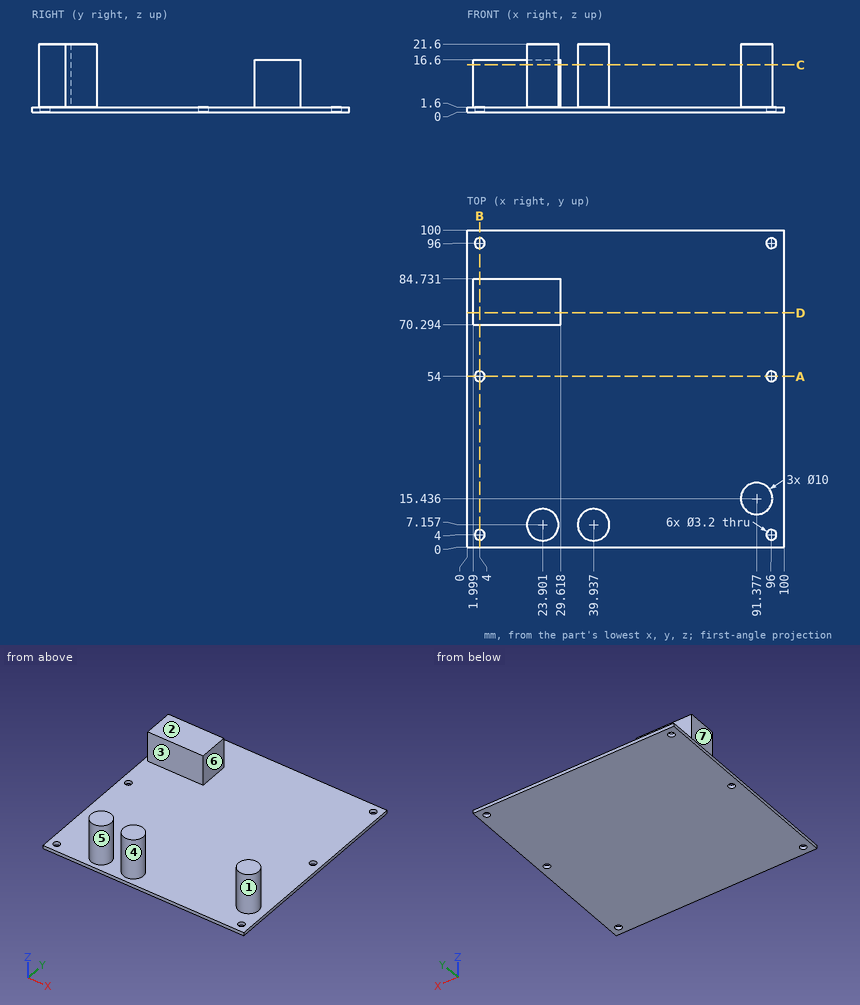
Study the drawing (mm; zero at the part's minimum x, y, z) and answer. A direction names the side the tool comes from. Round coordinates to 2 decimals unless told otherwise and drop trailing zeros. Write each loop counter-clockwise with the first axis right and the second up, starting at its lowest first coordinate (ties: lowest second). Pieces come first, ordered by that corner, then holes. Notation, with made-up numbers: (85, 68.25) - (131, 68.25) arc R3 ccw to (131, 73.25) - close; hole circle Ø8 at (-23, 49.5). An arc over 180 degrees is marked (long way). Return JSON: item names as keys, results as strings. Group by question number.
Q1. Find the intervals of material crossed by L1, parallel to Y at x = 96, z = 0.7; L2, parallel to Z at x = 7.5, y = 47; L3, parallel to Z at x = 21, y = 77, in increasing order.
Q2. Each of these flat-tipped pins is pushed along its axis until it touches: pin 1 Ø4 at (y, z) = (79.5, 5.5) entering from -X; pin 2 Ø12 at (x, z) = (31.5, 18.5) entering from -Y; pin 3 Ø4.5 at (x, z) = (12.5, 6) entering from +Y. Where does it stop, or does it pass through?
Q3. The part is cut by section D-D on y = 74. Write down the section's boundary in (x, z).
Q4. The part is cut by section A-A on y = 54. Write down the section's boundary in (x, z).
Q5. The mould has two halves that part along X. Classify the marked faces 4, 5, 6 and 7: released by +X, released by -X, zero draft, split by the parting line, or undercut.
Q6. The part is cut by section B-B on x = 4. Write down the section's boundary in (y, z).
Q7. The part is cut by section C-C on z = 15. Write down the section's boundary in (x, y).
Q8. For the marked faces 1, 2 and 3, determine the directions among +Z, -Z, +X, -X, +Y, -Y from which every point of the face is accessible in a straight line to the end or side of a thin tool.
Solved:
{
 "1": {"L1": "0 to 2.4, 5.6 to 52.4, 55.6 to 94.4, 97.6 to 100", "L2": "0 to 1.6", "L3": "0 to 16.6"},
 "2": {"pin 1": "x = 2", "pin 2": "y = 2.42", "pin 3": "y = 84.73"},
 "3": {"outline": "(0, 0) - (100, 0) - (100, 1.6) - (29.62, 1.6) - (29.62, 16.6) - (2, 16.6) - (2, 1.6) - (0, 1.6) - close"},
 "4": {"outline": "(0, 0) - (2.4, 0) - (2.4, 1.6) - (0, 1.6) - close; (5.6, 0) - (94.4, 0) - (94.4, 1.6) - (5.6, 1.6) - close; (97.6, 0) - (100, 0) - (100, 1.6) - (97.6, 1.6) - close"},
 "5": {"face 4": "undercut", "face 5": "undercut", "face 6": "released by +X", "face 7": "released by -X"},
 "6": {"outline": "(0, 0) - (2.4, 0) - (2.4, 1.6) - (0, 1.6) - close; (5.6, 0) - (52.4, 0) - (52.4, 1.6) - (5.6, 1.6) - close; (55.6, 0) - (94.4, 0) - (94.4, 1.6) - (84.73, 1.6) - (84.73, 16.6) - (70.29, 16.6) - (70.29, 1.6) - (55.6, 1.6) - close; (97.6, 0) - (100, 0) - (100, 1.6) - (97.6, 1.6) - close"},
 "7": {"outline": "(2, 70.29) - (29.62, 70.29) - (29.62, 84.73) - (2, 84.73) - close; circle Ø10 at (23.9, 7.16); circle Ø10 at (39.94, 7.16); circle Ø10 at (91.38, 15.44)"},
 "8": {"face 1": "+Z", "face 2": "+Z, +X, -X, +Y", "face 3": "+Z, +X, -X"}
}
